from build123d import *

# Parameters (mm, degrees)
PAD_DEPTH     = 10
SKETCH001_W   = 43
SKETCH001_H   = 18
SKETCH001_W_2 = 37
SKETCH001_H_2 = 12
PAD001_DEPTH  = 7.5
FILLET_R      = 5.99
FILLET001_R   = 2
FILLET002_R   = 2


with BuildPart() as part:
    # Sketch → Pad (new body)
    with BuildSketch(Plane.XZ):
        with BuildLine():
            ThreePointArc((3.68273, 0), (0, 7.75), (-3.68273, 0))
            Line((-3.68273, 0), (3.68273, 0))
        make_face()
    extrude(amount=PAD_DEPTH)

    # Sketch001 → Pad001 (join)
    with BuildSketch(Plane.XY):
        with Locations((0, 9)):
            Rectangle(SKETCH001_W, SKETCH001_H)
        with Locations((0, 9)):
            Rectangle(SKETCH001_W_2, SKETCH001_H_2, mode=Mode.SUBTRACT)
    extrude(amount=PAD001_DEPTH)

    # Fillet
    fillet_edges = [part.edges().sort_by_distance(p)[0] for p in [
        (-18.5, 15, 3.75),
        (-18.5, 3, 3.75),
        (18.5, 3, 3.75),
        (18.5, 15, 3.75),
    ]]
    fillet(fillet_edges, radius=FILLET_R)

    # Fillet001
    fillet001_edges = [part.edges().sort_by_distance(p)[0] for p in [
        (-21.5, 0, 3.75),
        (-21.5, 18, 3.75),
        (21.5, 18, 3.75),
        (21.5, 0, 3.75),
    ]]
    fillet(fillet001_edges, radius=FILLET001_R)

    # Fillet002
    fillet002_edges = [part.edges().sort_by_distance(p)[0] for p in [
        (0, -10, 7.75),
        (0, -10, 0),
    ]]
    fillet(fillet002_edges, radius=FILLET002_R)


solid = part.part
Design review of the part built by this model. Coordinates are the model's own, in mm. A direction names the side the tool comes from. Round coordinates to 2 decimals unless told otherwise and drop trailing zeros. Loops run counter-clockwise (first coordinate to the right, second up) from the corner with the lowest first, then second, coordinate; pieces in that order, holes last. Notation, with made-up numbers: (21, -33.5) - (76, -33.5) arc R28 ccw to (76, -11.5) - close; hole circle Ø11 at (41, 27.25). An arc over 180 degrees is marked (long way). One line per item, written item: value. Start each with the question number.
1) Insertion check: pin 1 Ø6 at (x, y) = (4, 4) entering from -Z; pin 2 Ø4 at (x, z) = (-7.5, 4) entering from -Y. Each pin has a flat end and moves straight along its axis. Give the tip position at first contact, or say it passes through.
2) Draft analysis for pull direction Y (two halves, no side actions). For faces 4 (the flat face through (0, 18, 4)), 5 (the flat face through (-21.5, 9, 4)), 6 (the flat face through (0, 3, 4)), 7 (the cylindrical face through (-16.7, 4.71, 3.8)), state which applies: +Y half, -Y half, draft (parallel to the pull), parting line (faces both ways), or undercut.
3) Consider section A-A on x = 0. Give the boundary of the cut face in (y, z).
4) Consider section B-B on y = 13.5. Give the boundary of the cut face in (x, z), then the cut area to 3 significant figures.
5) For faces 1 (the cylindrical face through (-16.7, 13.29, 3.8)), 2 (the cylindrical face through (0.15, -3.944, 7.748)), 3 (the cylindrical face through (-20.93, 17.4, 3.8)), list the 3-axis set-ups (+Z, -Z, +X, -X, +Y, -Y) from which the entire face can be reached by the end or side of a thin tool; tool diameter is ignored.
6) To check wall thickness, follow L1, parallel to Y at x = -11, z = 2.5; L2, parallel to Y at x = -1.5, z = 5.25; L3, parallel to Z at x = 1.5, y = -1.25. State the ranges of each line that lie inside material, in increasing order. Write a range as from..to.
7) Consider section C-C on x = 9. Give the boundary of the cut face in (y, z), then the cut area to 3 significant figures.
Reported:
1. pin 1: stops at z = 0
1. pin 2: stops at y = 0
2. face 4: +Y half
2. face 5: draft
2. face 6: undercut
2. face 7: undercut
3. outline: (-10, 2) arc R2 ccw to (-8, 0) - (3, 0) - (3, 7.5) - (0, 7.5) - (0, 7.75) - (-8, 7.75) arc R2 ccw to (-10, 5.75) - close; (15, 0) - (18, 0) - (18, 7.5) - (15, 7.5) - close
4. outline: (-21.5, 0) - (-16.47, 0) - (-16.47, 7.5) - (-21.5, 7.5) - close; (16.47, 0) - (21.5, 0) - (21.5, 7.5) - (16.47, 7.5) - close
4. area: 75.4 mm^2
5. face 1: +Z, -Z
5. face 2: -Y
5. face 3: +Z, -Z, -X, +Y
6. L1: y = 0..3, 15..18
6. L2: y = -10..3, 15..18
6. L3: z = 0..7.51
7. outline: (0, 0) - (3, 0) - (3, 7.5) - (0, 7.5) - close; (15, 0) - (18, 0) - (18, 7.5) - (15, 7.5) - close
7. area: 45.0 mm^2
